Input: part model. Units: mm. Frame: model coordinates. Face numbers are marked on the shaded views. A direction names the side the tool comes from. Coordinates: 2 decimals unless noted, no trailing zeros. Order: outer loops, then holes, each group sorted by start corner. A loop starts at its lowest first (then second) coordinate and runs counter-clockwise, first axis right, second up. Notation, with made-up numbers: (21.25, 52.5) -> (28.25, 52.5) arc R9 ccw to (28.25, 69.5) -> close; hole circle Ø8 at (38.5, 84). An arc over 180 degrees is marked (long way). One line per question, with ' | ' between items.
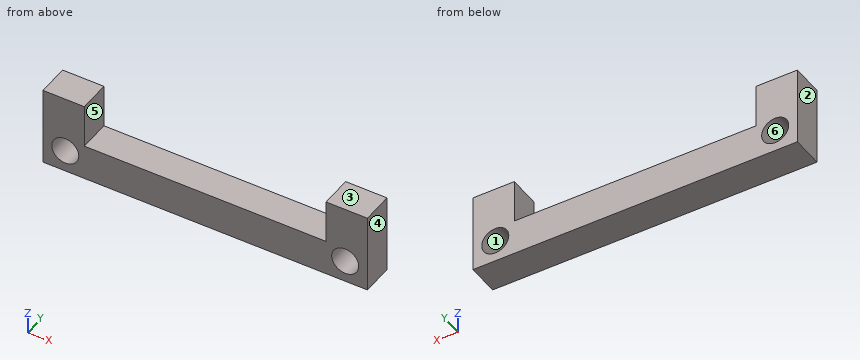
```python
from build123d import *

# Parameters (mm, degrees)
SKETCH1_R           = 4.25
BOSS_EXTRUDE1_DEPTH = 10


with BuildPart() as part:
    # Sketch1 → Boss-Extrude1 (new body)
    with BuildSketch(Plane(origin=(0, 0, 0), x_dir=(1, 0, 0), z_dir=(0, 1, 0))):
        Polygon((-51, 11.25), (51, 11.25), (51, 0), (51, -13.75), (38, -13.75), (38, 0), (-38, 0), (-38, -13.75), (-51, -13.75), align=None)
        with Locations(Location((-44, 4.25, 0), (0, 0, 270))):
            Circle(SKETCH1_R, mode=Mode.SUBTRACT)
        with Locations(Location((44, 4.25, 0), (0, 0, 90))):
            Circle(SKETCH1_R, mode=Mode.SUBTRACT)
    extrude(amount=BOSS_EXTRUDE1_DEPTH)


solid = part.part
```
1. Cut plane A-A, the plane z = 7.5. Return loops of the section in (x, y), and give its area (3 significant figures).
Recorded:
outline: (-51, 0) -> (-38, 0) -> (-38, 10) -> (-51, 10) -> close; (38, 0) -> (51, 0) -> (51, 10) -> (38, 10) -> close | area: 260 mm^2
2. Pin query (flat end, axial travel): pin 1 Ø1 at (x, y) = (21.5, 3.5) entering from +Z. Return the tip coordinate at first contact, or that it passes through.
Recorded:
pin 1: stops at z = 0
3. Mould query, pull axis X, two halves, no side actions, for the marked faces 1, 2, 3 and 4. Classes: released by +X, released by -X, zero draft, split by the parting line, or undercut.
Recorded:
face 1: undercut | face 2: released by -X | face 3: zero draft | face 4: released by +X
4. Cut plane D-D, the plane z = -7. Return loops of the section in (x, y).
Recorded:
outline: (-51, 0) -> (-47.24, 0) -> (-47.24, 10) -> (-51, 10) -> close; (-40.76, 0) -> (40.76, 0) -> (40.76, 10) -> (-40.76, 10) -> close; (47.24, 0) -> (51, 0) -> (51, 10) -> (47.24, 10) -> close
5. Cut plane C-C, the plane x = -44. Return loops of the section in (y, z), and give its area (3 significant figures).
Recorded:
outline: (0, -11.25) -> (10, -11.25) -> (10, -8.5) -> (0, -8.5) -> close; (0, 0) -> (10, 0) -> (10, 13.75) -> (0, 13.75) -> close | area: 165 mm^2
6. Access query for the marked faces 5 and 6. Directions: +Z, -Z, +X, -X, +Y, -Y. A direction counts if a zero-diameter tool reaches every point of the face in a straight line with its end or side. Return the directions, or none.
Recorded:
face 5: +Z, +Y, -Y | face 6: +Y, -Y
7. Ray query, line 1 (X direction, y = 2.75, z = -4.25); line 2 (X direction, y = 4, z = 4); line 3 (X direction, y = 8.25, z = -2.25). Return the intervals inside material, ascending. Write a range as [from, to].
Recorded:
line 1: x = [-51, -48.25], [-39.75, 39.75], [48.25, 51] | line 2: x = [-51, -38], [38, 51] | line 3: x = [-51, -47.75], [-40.25, 40.25], [47.75, 51]
8. Cut plane B-B, the plane y = 8.75. Return loops of the section in (x, z).
Recorded:
outline: (-51, -11.25) -> (51, -11.25) -> (51, 13.75) -> (38, 13.75) -> (38, 0) -> (-38, 0) -> (-38, 13.75) -> (-51, 13.75) -> close; hole circle Ø8.5 at (-44, -4.25); hole circle Ø8.5 at (44, -4.25)
